```python
from build123d import *

# Parameters (mm, degrees)
SKETCH1_R           = 4.75
BOSS_EXTRUDE1_DEPTH = 16.5
SKETCH2_R           = 1.95
BOSS_EXTRUDE2_DEPTH = 8.5
BOSS_EXTRUDE3_DEPTH = 1.05


with BuildPart() as part:
    # Sketch1 → Boss-Extrude1 (new body)
    with BuildSketch(Plane(origin=(0, 0, 0), x_dir=(1, 0, 0), z_dir=(0, 1, 0))):
        Circle(SKETCH1_R)
    extrude(amount=BOSS_EXTRUDE1_DEPTH)

    # Sketch2 → Boss-Extrude2 (add)
    with BuildSketch(Plane(origin=(0, 16.5, 0), x_dir=(1, 0, 0), z_dir=(0, 1, 0))):
        Circle(SKETCH2_R)
    extrude(amount=BOSS_EXTRUDE2_DEPTH)

    # Sketch3 → Boss-Extrude3 (add)
    with BuildSketch(Plane.XZ):
        with BuildLine():
            Line((-5.378429139, 1.15), (-4.645006983, 0.993181818))
            ThreePointArc((-4.645006983, 0.993181818), (-4.75, 0), (-4.645006983, -0.993181818))
            Line((-4.645006983, -0.993181818), (-5.378429139, -1.15))
            ThreePointArc((-5.378429139, -1.15), (-5.5, 0), (-5.378429139, 1.15))
        make_face()
        with BuildLine():
            Line((4.645006983, -0.993181818), (5.378429139, -1.15))
            ThreePointArc((5.378429139, -1.15), (5.5, 0), (5.378429139, 1.15))
            Line((5.378429139, 1.15), (4.645006983, 0.993181818))
            ThreePointArc((4.645006983, 0.993181818), (4.75, 0), (4.645006983, -0.993181818))
        make_face()
    extrude(amount=-BOSS_EXTRUDE3_DEPTH)


solid = part.part
```
Here's how the part is built. I have some questions about the finished solid (model axes, mm). A direction names the side the tool comes from. Give positions to 0.01 mm unless a question says otherwise; leave off trailing zeros. Loops run counter-clockwise (first coordinate to the right, second up) from the corner with the lowest first, then second, coordinate; pieces in that order, holes last. Notation, with made-up numbers: M 50,10.5 L 99,10.5 A25 cw 99,22.5 Z; hole C 6.5,79.5 d1. An arc over 180 degrees is marked long. Use one line per item in the form item = value. Start each with the question number.
Q1. Which directions (+Z, -Z, +X, -X, +Y, -Y) give clear straight access to the entire face, cutting with the end or side of a thin tool? Please do faces 1 (the flat face through (2, 16.5, 1)), 2 (the cylindrical face through (-5.5, 0.5, 0)).
Q2. If we section it at C-C (y = 4.5): Write out the boundary of the cut face in (x, z).
Q3. If we section it at D-D (y = 19.5): Write out the boundary of the cut face in (x, z).
Q4. If we section it at B-B (x = 0): Write out the boundary of the cut face in (y, z), then the cut area to 3 significant figures.
Q5. If we section it at A-A (z = 0): Write out the boundary of the cut face in (x, y).
Q6. I need wall thicknesses on line 1 along Y through (x, z) = (-1, -1.75); line 2 along X through (y, z) = (20.5, -1.75); line 3 along Z through (x, y) = (1.75, 12.5). Which ranges of each line are inside material? Lowest first, please.
Q7. Will these pins go through, and if not, where does the flat tip stop? pin 1 Ø1 at (x, y) = (2, 14.5) entering from +Z; pin 2 Ø5 at (y, z) = (14, -3.5) entering from -X; pin 3 Ø3 at (y, z) = (20.5, -0.5) entering from +X.
Taken from the geometry:
q1.face_1 = +Y
q1.face_2 = -X, +Y, -Y
q2.outline = C 0,0 d9.5
q3.outline = C 0,0 d3.9
q4.outline = M 0,-4.75 L 16.5,-4.75 L 16.5,-1.95 L 25,-1.95 L 25,1.95 L 16.5,1.95 L 16.5,4.75 L 0,4.75 Z
q4.area = 190 mm^2
q5.outline = M -5.5,0 L 5.5,0 L 5.5,1.05 L 4.75,1.05 L 4.75,16.5 L 1.95,16.5 L 1.95,25 L -1.95,25 L -1.95,16.5 L -4.75,16.5 L -4.75,1.05 L -5.5,1.05 Z
q6.line_1 = 0 to 16.5
q6.line_2 = -0.86 to 0.86
q6.line_3 = -4.42 to 4.42
q7.pin_1 = 4.51
q7.pin_2 = -4.64
q7.pin_3 = 1.95
